Model file for the job. Use its own axes, mm. A direction names the side the tool comes from. Coordinates: 2 decimals unless noted, no trailing zeros. Order: outer loops, then holes, each group sorted by start corner. A loop starts at its lowest first (then second) coordinate and runs counter-clockwise, first axis right, second up. Notation, with made-up numbers: (87, -32.5) -> (105, -32.5) arc R27 ccw to (105, -13.5) -> close; hole circle Ø10 at (54, 8). An arc over 180 degrees is marked (long way). Return JSON: item names as keys, results as strings. Group by question number.
1) Cut at D-D (y = 6). Write the cut outline in (x, z).
2) Probe line 1 (Y direction, x = 14.45, z = 7); line 2 (Z direction, x = 16.5, y = 3.5); line 3 (Y direction, x = 4.5, z = -4.75). List the from-to ranges inside material, lowest first.
3) Cut at C-C (x = 14.45). State how many separate pieces and enclosed holes the cut face has, and give its area (3 significant figures).
4) Pull direction X, two halves, no side cores. Call faces 5 (the flat face through (13, 4, 7.5)), 6 (the cylindrical face through (19.883, -0.205, 0.112)), 7 (the cylindrical face through (-22.63, -0.67, 8.71)): +X half, -X half, draft (parallel to the pull), parting line (faces both ways), or undercut.
5) Which spindle directions (+Z, -Z, +X, -X, +Y, -Y) get a long thin tool onto all of the face, cutting with end or side? Do faces 1 (the flat face through (13, 4, -7.5)), 2 (the cylindrical face through (19.344, 2.641, -7.007)), 3 (the cylindrical face through (23.79, -4.58, 8.7)), 4 (the flat face through (0, 0, 0)). Say none if no direction does.
6) Flat gauge pins, fed straight in: pin 1 (1.8 mm diameter, centred on x = 8, y = 5, fed in from -Z); pin 2 (8 mm diameter, centred on y = 4, z = 2, fed in from -X); pin 3 (5 mm diameter, centred on x = -0.5, z = 1, fed in from -Y). Where does each tip first touch, or does it go through?
from build123d import *

# Parameters (mm, degrees)
EXTRUDE_THIN1_DEPTH = 9
FILLET1_R           = 3
FILLET2_R           = 1
SKETCH2_R           = 1
EXTRUDE1_DEPTH      = 1


with BuildPart() as part:
    # Sketch1 → Extrude-Thin1 (new, symmetric)
    with BuildSketch(Plane.XY):
        with BuildLine():
            Line((-23.75, -5), (-20.6, -0.8))
            ThreePointArc((-20.6, -0.8), (-19.894427191, -0.211145618), (-19, 0))
            Line((-19, 0), (19, 0))
            ThreePointArc((19, 0), (19.894427191, -0.211145618), (20.6, -0.8))
            Line((20.6, -0.8), (28.25, -11))
            Line((28.25, -11), (29.85, -9.8))
            Line((29.85, -9.8), (22.2, 0.4))
            ThreePointArc((22.2, 0.4), (20.788854382, 1.577708764), (19, 2))
            Line((19, 2), (-19, 2))
            ThreePointArc((-19, 2), (-20.788854382, 1.577708764), (-22.2, 0.4))
            Line((-22.2, 0.4), (-25.35, -3.8))
            Line((-25.35, -3.8), (-23.75, -5))
        make_face()
    extrude(amount=EXTRUDE_THIN1_DEPTH, both=True)

    # Fillet1
    fillet1_edges = [part.edges().sort_by_distance(p)[0] for p in [
        (29.05, -10.4, -9),
        (-24.55, -4.4, -9),
        (29.05, -10.4, 9),
        (-24.55, -4.4, 9),
    ]]
    fillet(fillet1_edges, radius=FILLET1_R)

    # Fillet2
    fillet2_edges = [part.edges().sort_by_distance(p)[0] for p in [
        (-21.275, -1.7, 9),
        (20.788854382, 1.577708764, -9),
        (0, 0, -9),
        (-20.788854382, 1.577708764, -9),
        (-21.275, -1.7, -9),
        (-22.875, -0.5, -9),
        (-20.788854382, 1.577708764, 9),
        (0, 0, 9),
        (20.788854382, 1.577708764, 9),
        (-23.75, -5, 0),
        (-25.35, -3.8, 0),
        (-24.822792206, -3.097056275, -8.121320344),
        (-24.822792206, -3.097056275, 8.121320344),
        (0, 2, 9),
        (23.525, -4.7, 9),
        (25.125, -3.5, 9),
        (25.125, -3.5, -9),
        (23.525, -4.7, -9),
        (28.25, -11, 0),
        (27.722792206, -10.297056275, 8.121320344),
        (-22.875, -0.5, 9),
        (27.722792206, -10.297056275, -8.121320344),
        (29.85, -9.8, 0),
        (0, 2, -9),
    ]]
    fillet(fillet2_edges, radius=FILLET2_R - 0.0001)  # a hair under: the kernel refuses the full size

    # Sketch2 → Extrude1 (add)
    with BuildSketch(Plane.XY.offset(7.5)):
        with BuildLine():
            Line((2.45, 2), (13.5255002, 7.7734994))
            ThreePointArc((13.5255002, 7.7734994), (14.893058146, 7.950307535), (16.05, 7.2))
            Line((16.05, 7.2), (19.05, 3.2))
            ThreePointArc((19.05, 3.2), (19.347366596, 2.632455532), (19.45, 2))
            Line((19.45, 2), (19.45, 1.974606899))
            ThreePointArc((19.45, 1.974606899), (19.225357943, 1.993646679), (19, 2))
            Line((19, 2), (2.45, 2))
        make_face()
        with Locations((14.45, 6)):
            Circle(SKETCH2_R, mode=Mode.SUBTRACT)
    extrude1 = extrude(amount=-EXTRUDE1_DEPTH)

    # Mirror1: Extrude1 across plane
    add(extrude1.mirror(Plane.XY))


solid = part.part
Answers below:
{
 "1": {"outline": "(10.12, -7.5) -> (13.45, -7.5) -> (13.45, -6.5) -> (10.12, -6.5) -> close; (10.12, 6.5) -> (13.45, 6.5) -> (13.45, 7.5) -> (10.12, 7.5) -> close; (15.45, -7.5) -> (16.95, -7.5) -> (16.95, -6.5) -> (15.45, -6.5) -> close; (15.45, 6.5) -> (16.95, 6.5) -> (16.95, 7.5) -> (15.45, 7.5) -> close"},
 "2": {"line 1": "y = 0 to 5, 7 to 8", "line 2": "z = -7.5 to -6.5, 6.5 to 7.5", "line 3": "y = 0 to 2"},
 "3": {"separate pieces": "3", "enclosed holes": "0", "area": "43.1 mm^2"},
 "4": {"face 5": "draft", "face 6": "undercut", "face 7": "-X half"},
 "5": {"face 1": "-Z, +X, -X, +Y", "face 2": "+Z, -Z, +X, +Y", "face 3": "+Z, -Y", "face 4": "+Z, -Z, -Y"},
 "6": {"pin 1": "stops at z = -7.5", "pin 2": "stops at x = -22.5", "pin 3": "stops at y = 0"}
}
